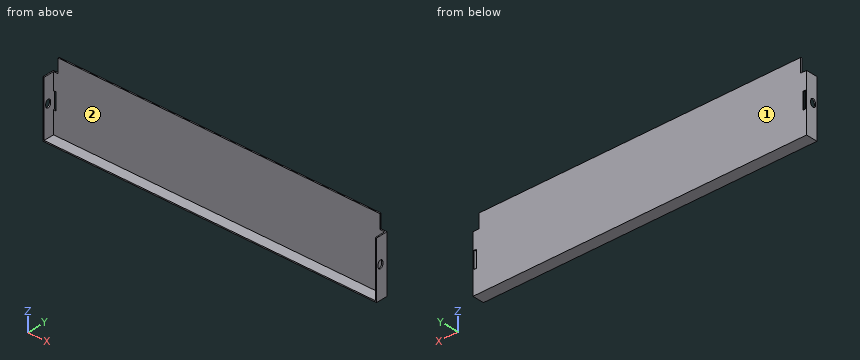
from build123d import *

# Parameters (mm, degrees)
SKETCH_1_W          = 2.2
SKETCH_1_H          = 14.5
EXTRUDE_1_DEPTH     = 1
EXTRUDE_2_DEPTH     = 9
CUT_EXTRUDE_1_DEPTH = 288.762488869


with BuildPart() as part:
    # Эскиз1 → Бобышка-Вытянуть1 (new body)
    with BuildSketch(Plane(origin=(0, 0, 0), x_dir=(1, 0, 0), z_dir=(0, 1, 0))):
        Polygon((138, -30.5), (138, -18.5), (143, -18.5), (143, 30.5), (-143, 30.5), (-143, -18.5), (-138, -18.5), (-138, -30.5), align=None)
        with Locations((140.9, 3.25)):
            Rectangle(SKETCH_1_W, SKETCH_1_H, mode=Mode.SUBTRACT)
        with Locations((-140.9, 3.25)):
            Rectangle(SKETCH_1_W, SKETCH_1_H, mode=Mode.SUBTRACT)
    extrude(amount=EXTRUDE_1_DEPTH)

    # Эскиз2 → Бобышка-Вытянуть2 (add)
    with BuildSketch(Plane.XZ):
        Polygon((-143, 18.5), (-143, -30.5), (143, -30.5), (143, 18.5), (142, 18.5), (142, -29.5), (-142, -29.5), (-142, 18.5), align=None)
    extrude(amount=EXTRUDE_2_DEPTH)

    # Эскиз3 → Вырез-Вытянуть1 (cut, through all)
    with BuildSketch(Plane(origin=(143, 0, 0), x_dir=(0, 0, -1), z_dir=(1, 0, 0))):
        with BuildLine():
            Line((2.2, -3), (4.3, -3))
            ThreePointArc((4.3, -3), (6.55, -5.25), (4.3, -7.5))
            Line((4.3, -7.5), (2.2, -7.5))
            ThreePointArc((2.2, -7.5), (-0.05, -5.25), (2.2, -3))
        make_face()
    extrude(amount=-CUT_EXTRUDE_1_DEPTH, mode=Mode.SUBTRACT)


solid = part.part
Check sheet for the modelled part. Datum: model origin and axes. Units: mm. Face numbers are marked on the shaded views. Give positions to 0.01 mm unless a question says otherwise; leave off trailing zeros. Write each loop counter-clockwise with the first axis right and the second up, starting at its lowest first coordinate (ties: lowest second). Pieces come first, ordered by that corner, then holes. Notation, with made-up numbers: M 67.25,21.25 L 73.25,21.25 A17 ccw 73.25,40.25 Z; hole C -9,23.25 d11. An arc over 180 degrees is marked long. Use one line per item in the form item = value.
(1) Section check C-C on x = 75. Record the boundary of the cut face in (y, z).
Answer block:
outline = M -9,-30.5 L 1,-30.5 L 1,30.5 L 0,30.5 L 0,-29.5 L -9,-29.5 Z
(2) Depth check by flat-ended pin: P1, Ø1.1, axis at y = 0.5, z = 26.5, coming from the +X side; P2, Ø1.1, axis at y = 0.5, z = 27, coming from the -X side; P3, Ø1, axis at x = -18, z = 23.5, coming from the -Y side. Enter the tip coordinate at first touch or a pass-through.
Answer block:
P1 = 138
P2 = -138
P3 = 0
(3) Section check B-B on z = 10.5. Record the boundary of the cut face in (x, y).
Answer block:
outline = M -143,-9 L -142,-9 L -142,0 L 142,0 L 142,-9 L 143,-9 L 143,1 L -143,1 Z
(4) Draft check along X on the marked faces 1 and 2. Enter one of: pulls with the +X half, pulls with the -X half, needs draft (parallel to the pull), parting line crosses it, or undercut.
Answer block:
face_1 = needs draft
face_2 = undercut
(5) Material ranges on line 1 along X through (y, z) = (-7.75, -12); line 2 along Z through (x, y) = (-110, -0.5); line 3 along Y through (x, z) = (103.5, -11.5), recorded low to high.
Answer block:
line_1 = -143 to -142, 142 to 143
line_2 = -30.5 to -29.5
line_3 = 0 to 1
(6) Section check A-A on y = -5.25. Record the boundary of the cut face in (x, z), plus the area to 3 significant figures.
Answer block:
outline = M -143,-30.5 L 143,-30.5 L 143,-6.55 L 142,-6.55 L 142,-29.5 L -142,-29.5 L -142,-6.55 L -143,-6.55 Z; M -143,0.05 L -142,0.05 L -142,18.5 L -143,18.5 Z; M 142,0.05 L 143,0.05 L 143,18.5 L 142,18.5 Z
area = 369 mm2
